from build123d import *

# Parameters (mm, degrees)
SKETCH2_W          = 36
SKETCH2_H          = 8
CUT_EXTRUDE2_DEPTH = 252.956841542
SKETCH3_W          = 30
SKETCH3_H          = 8
CUT_EXTRUDE3_DEPTH = 253.227080227
FILLET1_R          = 1
CHAMFER1_SIZE      = 1


with BuildPart() as part:
    # Sketch1 → Revolve1 (revolve)
    with BuildSketch(Plane.XY, mode=Mode.PRIVATE) as revolve1_sk:
        Polygon((0, 0), (0, 12.5), (50, 12.5), (50, 15), (80, 15), (80, 17.5), (120, 17.5), (120, 15), (250, 15), (250, 0), align=None)
    revolve(revolve1_sk.sketch.rotate(Axis((0, 0, 0), (1, 0, 0)), 90), axis=Axis((0, 0, 0), (1, 0, 0)))

    # Sketch2 → Cut-Extrude2 (cut, through all)
    with BuildSketch(Plane(origin=(0, 8.5, 0), x_dir=(1, 0, 0), z_dir=(0, 1, 0))):
        with Locations((25, 0)):
            Rectangle(SKETCH2_W, SKETCH2_H)
    extrude(amount=CUT_EXTRUDE2_DEPTH, mode=Mode.SUBTRACT)

    # Sketch3 → Cut-Extrude3 (cut, through all)
    with BuildSketch(Plane(origin=(0, 11, 0), x_dir=(1, 0, 0), z_dir=(0, 1, 0))):
        with Locations((230, 0)):
            Rectangle(SKETCH3_W, SKETCH3_H)
    extrude(amount=CUT_EXTRUDE3_DEPTH, mode=Mode.SUBTRACT)

    # Fillet1
    fillet1_edges = [part.edges().sort_by_distance(p)[0] for p in [
        (80, 0, -15),
        (50, 0, -12.5),
        (120, 0, -15),
    ]]
    fillet(fillet1_edges, radius=FILLET1_R)

    # Chamfer1
    chamfer1_edges = [part.edges().sort_by_distance(p)[0] for p in [
        (0, 0, -12.5),
        (250, 0, -15),
    ]]
    chamfer(chamfer1_edges, length=CHAMFER1_SIZE)


solid = part.part
Geometry check sheet. Reference: the model listing, model coordinates, mm. A direction names the side the tool comes from. Give positions to 0.01 mm unless a question says otherwise; leave off trailing zeros. Order: outer loops, then holes, each group sorted by start corner. A loop starts at its lowest first (then second) coordinate and runs counter-clockwise, first axis right, second up.
1. Depth check by flat-ended pin: pin 1 (1.5 mm diameter, centred on x = 107.5, y = -8.5, fed in from -Z); pin 2 (1.7 mm diameter, centred on x = 23, y = 10.5, fed in from -Z); pin 3 (1 mm diameter, centred on x = 233.5, y = 12.5, fed in from -Z); pin 4 (3 mm diameter, centred on y = 9.5, z = 0, fed in from -X). Enter the tip coordinate at first touch or a pass-through.
Completed:
pin 1: stops at z = -15.69
pin 2: stops at z = -7.95
pin 3: stops at z = -9
pin 4: stops at x = 0
2. Sectioned sample at B-B (y = 0). Record the boundary of the cut face in (x, z).
Completed:
outline: (0, -11.5) - (1, -12.5) - (49, -12.5) arc R1 cw to (50, -13.5) - (50, -15) - (79, -15) arc R1 cw to (80, -16) - (80, -17.5) - (120, -17.5) - (120, -16) arc R1 cw to (121, -15) - (249, -15) - (250, -14) - (250, 14) - (249, 15) - (121, 15) arc R1 cw to (120, 16) - (120, 17.5) - (80, 17.5) - (80, 16) arc R1 cw to (79, 15) - (50, 15) - (50, 13.5) arc R1 cw to (49, 12.5) - (1, 12.5) - (0, 11.5) - close
3. Draft check along Z on faces 6 (the face through (250, 0, 0)), 7 (the face through (43, 10, 0)), 8 (the face through (185.9, -12.65, 8.06)), 9 (the face through (230, 11, 0)). Enter one of: pulls with the +Z half, pulls with the -Z half, needs draft (parallel to the pull), parting line crosses it, or undercut.
Completed:
face 6: needs draft
face 7: undercut
face 8: parting line crosses it
face 9: undercut
4. Access from +Z, -Z, +X, -X, +Y, -Y to the whole of each face (thin tool, end or side, straight path). Record for faces 1 (the face through (25.336, -12.394, -1.627)), 2 (the face through (215, 13, 0)), 3 (the face through (0, 0, 0)), 4 (the face through (100.28, 17.084, -3.794)), 5 (the face through (120, 14.2, 7.7)).
Completed:
face 1: -X
face 2: +Y
face 3: +Z, -Z, -X, +Y, -Y
face 4: +X, -X
face 5: +X
5. Scan lines: line 1 (Z direction, x = 108, y = 9); line 2 (X direction, y = -13.5, z = -9); line 3 (Z direction, x = 138, y = -6.5). Record each from-to range of solid material in increasing order.
Completed:
line 1: z = -15.01 to 15.01
line 2: x = 80 to 120
line 3: z = -13.52 to 13.52
6. Sectioned sample at D-D (x = 38). Record the boundary of the cut face in (y, z).
Completed:
outline: (8.5, -4) - (8.5, 4) - (11.84, 4) arc R12.5 ccw (long way) to (11.84, -4) - close
7. Sectioned sample at C-C (x = 159.5). Record the boundary of the cut face in (y, z), then the cut area to 3 significant figures.
Completed:
outline: circle Ø30 at (0, 0)
area: 707 mm2
